Input: part model. Units: mm. Frame: model coordinates. A direction names the side the tool comes from. Coordinates: 2 decimals unless noted, no trailing zeros. Order: outer loops, then holes, each group sorted by start corner. A loop starts at its lowest first (then second) coordinate and runs counter-clockwise, first axis right, second up.
from build123d import *

# Parameters (mm, degrees)
SKETCH_1_R               = 14
EXTRUDE_1_DEPTH          = 10
EXTRUDE_2_DEPTH          = 10
PATTERN_CIRCULAR_1_COUNT = 8
CUT_EXTRUDE_2_DEPTH      = 8
SKETCH_8_R               = 1.575
EXTRUDE_5_DEPTH          = 15


with BuildPart() as part:
    # ｽｹｯﾁ1 → ﾎﾞｽ - 押し出し1 (new body)
    with BuildSketch(Plane(origin=(0, 0, 0), x_dir=(1, 0, 0), z_dir=(0, 1, 0))):
        with Locations(Location((0, 0, 0), (0, 0, 270))):
            Circle(SKETCH_1_R)
    extrude(amount=EXTRUDE_1_DEPTH)

    # ｽｹｯﾁ3 → ﾎﾞｽ - 押し出し2 (add)
    with BuildSketch(Plane(origin=(0, 0, 0), x_dir=(1, 0, 0), z_dir=(0, 1, 0))):
        with BuildLine():
            ThreePointArc((0.670662773, 13.983926896), (-2.731264508, 13.730993926), (-5.971028752, 12.662812312))
            add(Edge.make_bspline(
                [(-5.528304984, 17.130027554), (-5.669447216, 16.763315044), (-5.860218101, 16.179410176), (-6.038366418, 15.38918786), (-6.12675066, 14.806480124), (-6.167823232, 14.2902167), (-6.171562682, 13.84380553), (-6.148097009, 13.46960438), (-6.10787192, 13.168784501), (-6.053435711, 12.906118131), (-6.005913858, 12.745636704), (-5.971028752, 12.662812312)],
                knots=[0, 0, 0, 0, 0.257950131, 0.40241706, 0.531259136, 0.64447636, 0.742068735, 0.824036262, 0.890378946, 0.941096793, 1, 1, 1, 1], degree=3))
            ThreePointArc((-5.528304984, 17.130027554), (-3.511625796, 17.654135047), (-1.447889917, 17.941672575))
            add(Edge.make_bspline(
                [(-1.447889917, 17.941672575), (-1.177156696, 17.656887186), (-0.77745666, 17.190434286), (-0.310464088, 16.528538472), (-0.0058151, 16.024009907), (0.229696468, 15.562762489), (0.403985429, 15.151763371), (0.525506554, 14.797066663), (0.603462201, 14.50375186), (0.65368777, 14.240247941), (0.671196886, 14.073796609), (0.670662773, 13.983926896)],
                knots=[0, 0, 0, 0, 0.257950131, 0.40241706, 0.531259136, 0.64447636, 0.742068735, 0.824036262, 0.890378946, 0.941096793, 1, 1, 1, 1], degree=3))
        make_face()
    extrude_2 = extrude(amount=EXTRUDE_2_DEPTH)

    # 円形ﾊﾟﾀｰﾝ1: ﾎﾞｽ - 押し出し2 ×8 about axis
    pattern_circular_1_axis = Axis((0, 10, 0), (0, 1, 0))
    for i in range(1, PATTERN_CIRCULAR_1_COUNT):
        add(extrude_2.rotate(pattern_circular_1_axis, i * 360 / PATTERN_CIRCULAR_1_COUNT))

    # ｽｹｯﾁ6 → ｶｯﾄ - 押し出し2 (cut)
    with BuildSketch(Plane(origin=(0, 10, 0), x_dir=(1, 0, 0), z_dir=(0, 1, 0))):
        Polygon((0, 5.773502692), (-5, 2.886751346), (-5, -2.886751346), (0, -5.773502692), (5, -2.886751346), (5, 2.886751346), align=None)
    extrude(amount=-CUT_EXTRUDE_2_DEPTH, mode=Mode.SUBTRACT)

    # ｽｹｯﾁ8 → ﾎﾞｽ - 押し出し5 (add)
    with BuildSketch(Plane(origin=(0, 2, 0), x_dir=(1, 0, 0), z_dir=(0, 1, 0))):
        with Locations(Location((0, 0, 0), (0, 0, 270))):
            Circle(SKETCH_8_R)
    extrude(amount=EXTRUDE_5_DEPTH)


solid = part.part
Item 1: Cut plane A-A on y = 6. Count the separate pieces of the cut face and the enclosed holes in it, then the cut area to 3 significant figures.
Response values:
separate pieces: 2
enclosed holes: 1
area: 730 mm2
Item 2: Cut plane B-B on x = 4. Return loops of the section in (y, z), then the cut area to 3 significant figures.
Response values:
outline: (0, -13.42) - (10, -13.42) - (10, -3.46) - (2, -3.46) - (2, 3.46) - (10, 3.46) - (10, 17.55) - (0, 17.55) - close
area: 254 mm2
Item 3: Cut plane C-C on y = 14.25. Return loops of the section in (x, z) (3 decimals).
Response values:
outline: circle Ø3.15 at (0, 0)
Item 4: Pin query (flat end, axial travel): pin 1 Ø3 at (y, z) = (8, 0.5) entering from +X; pin 2 Ø4 at (x, y) = (3.5, 8) entering from +Z; pin 3 Ø10 at (y, z) = (14.5, 13) entering from +X. Return the tip coordinate at first contact, or that it passes through.
Response values:
pin 1: stops at x = 17.44
pin 2: stops at z = 17.94
pin 3: stops at x = 14.38
Item 5: Draft query along X for faces 6 (the face through (3.54, 4.93, 17.65)), 7 (the face through (-0.96, 9.4, -1.25)), 8 (the face through (-2.535, 6.056, 4.31)), 9 (the face through (0, 17, 0)). Return one class per face: pulls with the +X half, pulls with the -X half, needs draft (parallel to the pull), parting line crosses it, or undercut.
Response values:
face 6: pulls with the +X half
face 7: undercut
face 8: undercut
face 9: needs draft
Item 6: Access query for faces 1 (the face through (2.76, 4.93, -13.725)), 2 (the face through (5, 6, 0)), 3 (the face through (-17.65, 4.93, 3.54)), 4 (the face through (-2.76, 4.93, 13.725)), 5 (the face through (13.725, 4.93, 2.76)). Directions: +Z, -Z, +X, -X, +Y, -Y. A direction counts if a zero-diameter tool reaches every point of the face in a straight line with its end or side. Return the directions, or none.
Response values:
face 1: -Z, +Y, -Y
face 2: +Y
face 3: +Z, -X, +Y, -Y
face 4: +Z, +Y, -Y
face 5: +X, +Y, -Y
Item 7: Ray query, probe 1 along Y at (x, z) = (-10.5, -1); probe 2 along X at (y, z) = (7.5, 10.5); probe 3 along Y at (x, z) = (0, -3). Return the intervals inside material, ascending.
Response values:
probe 1: y = 0 to 10
probe 2: x = -11.03 to 9.26, 9.57 to 14.62
probe 3: y = 0 to 2
